Autodesk Inventor part; units mm, degrees
ref_plane "YZ Plane" through (0, 0, 0) normal (1, 0, 0) x (0, 1, 0)
ref_plane "XZ Plane" through (0, 0, 0) normal (0, 1, 0) x (-1, 0, 0)
ref_plane "XY Plane" through (0, 0, 0) normal (0, 0, 1) x (1, 0, 0)
sketch "Sketch1" plane through (0, 0, 0) normal (0, 0, 1) x (1, 0, 0)
  line L0 (-10.9985, 0) -> (-5.4993, 9.525)
  line L1 (-5.4993, 9.525) -> (5.4993, 9.525)
  line L2 (5.4993, 9.525) -> (10.9985, 0)
  line L3 (10.9985, 0) -> (5.4993, -9.525)
  line L4 (5.4993, -9.525) -> (-5.4993, -9.525)
  line L5 (-5.4993, -9.525) -> (-10.9985, 0)
  point P0 (0, 0)
  point P1 (0, 0)
  dimension "d0" = 19.05
extrude "Extrusion1" add sketch "Sketch1" along normal blind 12.7
sketch "Sketch2" plane through (0, 0, 12.7) normal (0, 0, 1) x (1, 0, 0)
  circle A0 centre (0, 0) radius 6.35
  dimension "d3" = 12.7
extrude "Extrusion2" cut sketch "Sketch2" against normal blind 12.7
thread "Thread1"
fillet "Fillet1" radius 3.175 6 edges at (0, 9.525, 12.7) (8.2489, 4.7625, 12.7) (8.2489, -4.7625, 12.7) (0, -9.525, 12.7) (-8.2489, -4.7625, 12.7) (-8.2489, 4.7625, 12.7)
properties part number "LucasCharles part 5 nut final" material "Stainless Steel, Austenitic"
Part model, mm, in its own coordinate system. Coordinates: 2 decimals unless noted, no trailing zeros. Return JSON: item names as keys, results as strings. Group by question number.
Item 1: Drill centre lines: probe 1 along Y at (x, z) = (0, 9.5) (3 decimals); probe 2 along Y at (x, z) = (-3.5, 10.5); probe 3 along X at (y, z) = (2.25, 6). Where is each one in solid material? Low to high. Write a range as from..to.
Item 2: Pin check, flat tips, straight feed: pin 1 (1 mm diameter, centred on x = 4.5, z = 11, fed in from -Y); pin 2 (3 mm diameter, centred on x = -6.5, y = -3, fed in from +Z); pin 3 (6 mm diameter, centred on y = 3.5, z = 9, fed in from +X). Stop position of each tip, or through.
Item 3: Pull direction Y, two halves, no side cores. Call faces 1 (the face through (8.287, -4.696, 4.696)), 2 (the face through (0, 9.525, 5)), 3 (the face through (-1.38, -6.2, 6.44)): pulls with the +Y half, pulls with the -Y half, needs draft (parallel to the pull), parting line crosses it, or undercut.
Check values:
{
 "1": {"probe 1": "y = -9.525..-6.35, 6.35..9.525", "probe 2": "y = -9.37..-5.3, 5.3..9.37", "probe 3": "x = -9.7..-5.94, 5.94..9.7"},
 "2": {"pin 1": "stops at y = -9.37", "pin 2": "stops at z = 12.7", "pin 3": "stops at x = 10.71"},
 "3": {"face 1": "pulls with the -Y half", "face 2": "pulls with the +Y half", "face 3": "undercut"}
}
